The figure shows three views and two pictorial views of one solid part (mm, origin at its lowest corner). Answer the questions. A direction names the side the tool comes from. Give positions to 0.01 mm unless a question says otherwise; leave off trailing zeros. Write each loop counter-clockwise with the first axis right and the second up, starting at its lowest first coordinate (ties: lowest second). Pieces come first, ordered by that corner, then holes. Notation, with made-up numbers: (-2, 47) -> (7, 47) arc R27 cw to (7, 72) -> close; hole circle Ø4 at (-7.5, -2). An arc over 180 degrees is marked (long way). Answer as CSV lines item,"result". Start each with the question number.
1. A tool of negligible diameter and unlimited length cuts with its end or side. For the marked faces 4, 5 and 6, from which of +Z, -Z, +X, -X, +Y, -Y can it reach the whole face along a straight path? Write none if from no direction.
2. The part is cut by section C-C, the plane x = 7.5. Determine the outline of the cut face in (y, z), and give its area (3 significant figures).
3. The part is cut by section D-D, the plane z = 5. Determine the outline of the cut face in (x, y), and give its area (3 significant figures).
4. Find the intervals of material crossed by line 1 (Z direction, x = 42, y = 3.5); line 2 (X direction, y = 3.5, z = 28); line 3 (X direction, y = 6.5, z = 10), in increasing order.
5. The part is cut by section B-B, the plane y = 7.75. Determine the outline of the cut face in (x, z).
6. Given pin 1 (1.5 mm diameter, centred on x = 13.5, z = 30, fed in from +Y); pin 2 (12.5 mm diameter, centred on y = 15, z = 29.5, fed in from +X); pin 3 (6 mm diameter, centred on x = 14.5, y = 21.5, fed in from -Z); pin 4 (10 mm diameter, centred on y = 4, z = 4, fed in from +X), each flat-ended and moving along its own axis, determine where each tip first touches the part or whether it passes through.
7. For a pull along X with two mould halves and no side action, classify the marked faces 1, 2 and 3 as pulls with the +X half, pulls with the -X half, needs draft (parallel to the pull), parting line crosses it, or undercut.
8. The part is cut by section A-A, the plane z = 17. Determine the outline of the cut face in (x, y), and give its area (3 significant figures).
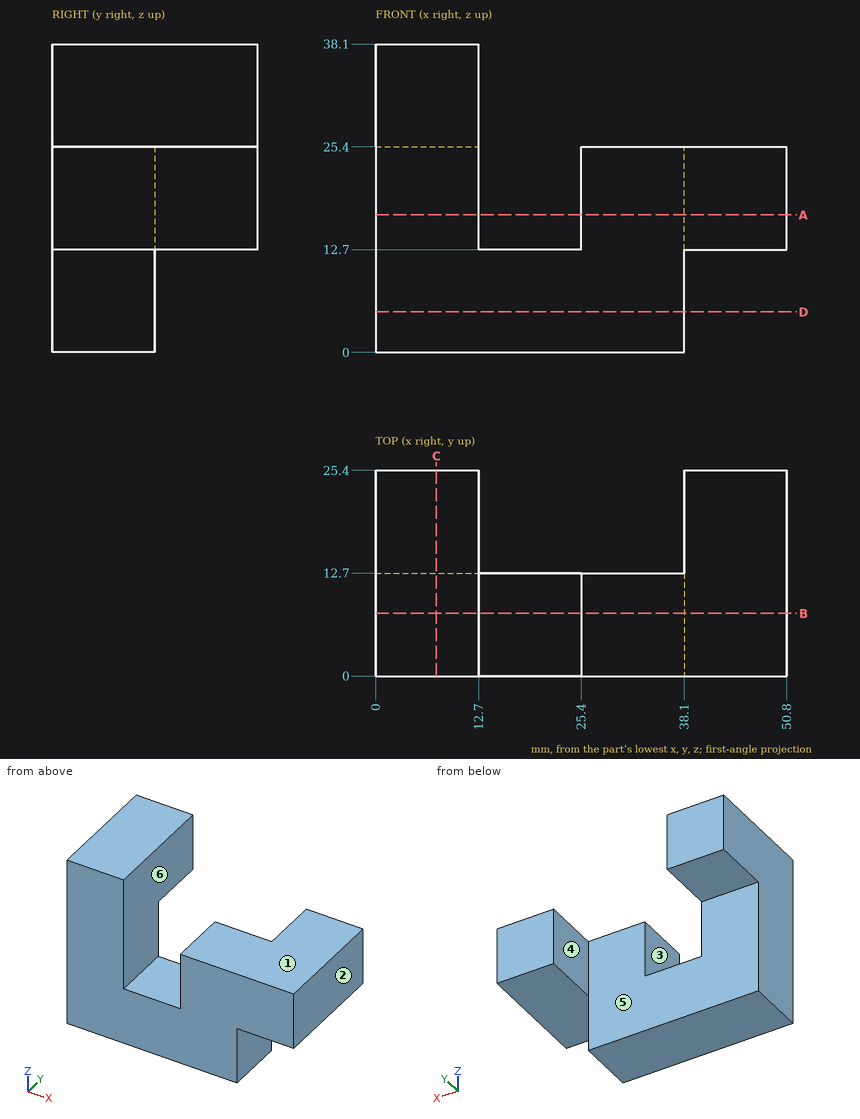
Results found:
1,face 4,"+Z, -Z, -X, +Y"
1,face 5,"-Z, -X, +Y"
1,face 6,"+Z, +Y, -Y"
2,outline,"(0, 0) -> (12.7, 0) -> (12.7, 25.4) -> (25.4, 25.4) -> (25.4, 38.1) -> (0, 38.1) -> close"
2,area,"645 mm²"
3,outline,"(0, 0) -> (38.1, 0) -> (38.1, 12.7) -> (0, 12.7) -> close"
3,area,"484 mm²"
4,line 1,"z = 12.7 to 25.4"
4,line 2,"x = 0 to 12.7"
4,line 3,"x = 0 to 38.1"
5,outline,"(0, 0) -> (38.1, 0) -> (38.1, 12.7) -> (50.8, 12.7) -> (50.8, 25.4) -> (25.4, 25.4) -> (25.4, 12.7) -> (12.7, 12.7) -> (12.7, 38.1) -> (0, 38.1) -> close"
6,pin 1,"passes through"
6,pin 2,"stops at x = 50.8"
6,pin 3,"stops at z = 25.4"
6,pin 4,"stops at x = 38.1"
7,face 1,"needs draft"
7,face 2,"pulls with the +X half"
7,face 3,"undercut"
8,outline,"(0, 0) -> (12.7, 0) -> (12.7, 12.7) -> (0, 12.7) -> close; (25.4, 0) -> (50.8, 0) -> (50.8, 25.4) -> (38.1, 25.4) -> (38.1, 12.7) -> (25.4, 12.7) -> close"
8,area,"645 mm²"
